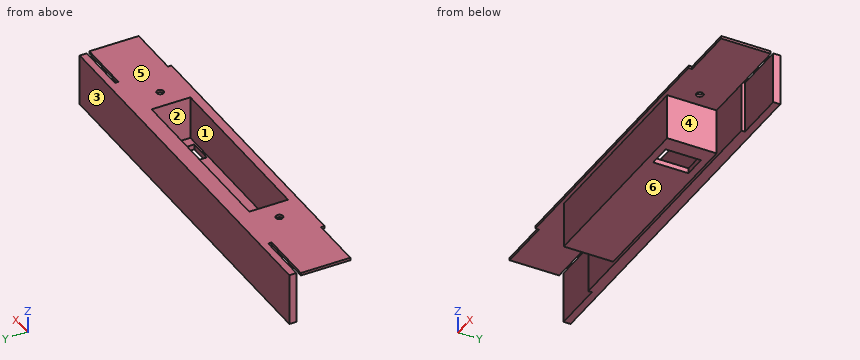
Autodesk Inventor part; units mm, degrees
ref_plane "YZ Plane" through (0, 0, 0) normal (1, 0, 0) x (0, 1, 0)
ref_plane "XZ Plane" through (0, 0, 0) normal (0, 1, 0) x (-1, 0, 0)
ref_plane "XY Plane" through (0, 0, 0) normal (0, 0, 1) x (1, 0, 0)
sketch "Эскиз1" plane through (0, 0, 0) normal (0, 0, 1) x (1, 0, 0)
  line L0 (-54, -14) -> (54, -14)
  line L1 (54, -14) -> (54, 14)
  line L2 (54, 14) -> (-54, 14)
  line L3 (-54, 14) -> (-54, -14)
  line L4 (-54, -14) -> (54, 14) construction
  line L5 (54, -14) -> (-54, 14) construction
  point P0 (0, 0)
  dimension "d0" = 108
  dimension "d1" = 28
extrude "Выдавливание1" add sketch "Эскиз1" along normal blind 27.5
sketch "Эскиз2" plane through (0, 0, 27.5) normal (0, 0, 1) x (1, 0, 0)
  line L0 (-51, -11) -> (51, -11)
  line L1 (51, -11) -> (51, 11)
  line L2 (51, 11) -> (-51, 11)
  line L3 (-51, 11) -> (-51, -11)
  line L4 (-51, -11) -> (51, 11) construction
  line L5 (51, -11) -> (-51, 11) construction
  line L6 (54, 14) -> (-54, 14)
  line L7 (54, -14) -> (54, 14)
  point P0 (0, 0)
  dimension "d4" = 3
  dimension "d5" = 3
extrude "Выдавливание2" cut sketch "Эскиз2" against normal blind 24.5
sketch "Эскиз3" plane through (54, -14, 0) normal (1, 0, 0) x (0, 0, -1)
  line L0 (0, 28) -> (-27.5, 28)
  line L1 (0, 0) -> (-27.5, 0)
  line L2 (-27.5, 28) -> (-26, 28)
  line L3 (-26, 28) -> (-26, 0)
  line L4 (-26, 0) -> (-27.5, 0)
  line L5 (-27.5, 0) -> (-27.5, 28)
  point P0 (0, 14)
  dimension "d8" = 1.5
extrude "Выдавливание3" add sketch "Эскиз3" along normal blind 50
mirror "Зеркальное отражение1" about plane through (0, 0, 0) normal (1, 0, 0) of "Выдавливание3"
move faces "Перенос1" translate (6.5, 0, 0) faces at (104, 4.6667, 27)
move faces "Перенос2" translate (-6.5, 0, 0) faces at (-104, 4.6667, 27)
sketch "Эскиз7" plane through (-54, -14, 0) normal (0, -1, 0) x (1, 0, 0)
  line L0 (-56.5, 27.5) -> (164.5, 27.5)
  line L1 (0, 26) -> (-56.5, 26)
  line L2 (134, 27.5) -> (-26, 27.5)
  line L3 (-26, 27.5) -> (-26, 26)
  line L4 (-26, 26) -> (134, 26)
  line L5 (134, 26) -> (134, 27.5)
  line L6 (0, 0) -> (108, 0)
  point P0 (54, 0)
  point P1 (-26, 26.75)
  point P2 (54, 0)
  dimension "d29" = 160
  dimension "d30" = 80
extrude "Выдавливание7" add sketch "Эскиз7" along normal blind 2
sketch "Эскиз8" plane through (-54, 14, 0) normal (0, 1, 0) x (1, 0, 0)
  line L0 (-56.5, -27.5) -> (164.5, -27.5)
  line L1 (-26, -27.5) -> (134, -27.5)
  line L2 (134, -27.5) -> (134, 2)
  line L3 (134, 2) -> (-26, 2)
  line L4 (-26, 2) -> (-26, -27.5)
  line L5 (108, 0) -> (0, 0)
  point P0 (54, 0)
  point P1 (54, 0)
  dimension "d33" = 160
  dimension "d34" = 80
  dimension "d35" = 29.5
extrude "Выдавливание8" add sketch "Эскиз8" along normal blind 6
sketch "Эскиз9" plane through (80, 14, 26) normal (1, 0, 0) x (0, 0, -1)
  line L0 (28, 0) -> (28, 6)
  line L1 (28, 6) -> (-1.5, 6)
  line L2 (-1.5, 6) -> (-1.5, 2)
  line L3 (-1.5, 2) -> (28, 2)
  line L4 (28, 2) -> (28, 6)
  point P0 (26, -14)
  dimension "d38" = 4
extrude "Выдавливание9" add sketch "Эскиз9" along normal blind 29.5
mirror "Зеркальное отражение3" about plane through (0, 0, 0) normal (1, 0, 0) of "Выдавливание9"
sketch "Эскиз10" plane through (0, 0, 27.5) normal (0, 0, 1) x (1, 0, 0)
  circle A0 centre (-62.25, 0) radius 2
  circle A1 centre (62.25, 0) radius 2
  point P0 (0, 0)
extrude "Выдавливание10" cut sketch "Эскиз10" against normal through all
sketch "Эскиз11" plane through (0, 0, 3) normal (0, 0, 1) x (1, 0, 0)
  line L0 (32, -10) -> (45, -10)
  line L1 (45, -10) -> (45, 10)
  line L2 (45, 10) -> (32, 10)
  line L3 (32, 10) -> (32, -10)
  line L4 (32, -10) -> (45, 10) construction
  line L5 (45, -10) -> (32, 10) construction
  line L6 (51, 11) -> (51, -11)
  point P0 (0, 0)
  point P1 (38.5, 0)
  dimension "d43" = 13
  dimension "d44" = 20
  dimension "d45" = 6
extrude "Выдавливание11" cut sketch "Эскиз11" against normal through all
properties part number "000.009 - Короб" material "Пластик АБС"
Check sheet for the modelled part. Datum: model origin and axes. Units: mm. Face numbers are marked on the shaded views. A direction names the side the tool comes from. Give positions to 0.01 mm unless a question says otherwise; leave off trailing zeros. Order: outer loops, then holes, each group sorted by start corner. A loop starts at its lowest first (then second) coordinate and runs counter-clockwise, first axis right, second up. Notation, with made-up numbers: (75, -15) -> (105, -15) arc R21 cw to (105, 24) -> close; hole circle Ø5 at (84.5, 2.25). An arc over 180 degrees is marked (long way). Use CSV: the item, a comma, the result in double quotes. Start each with the question number.
1) Material ranges on line 1 (Y direction, x = 39, z = 16.5); line 2 (Y direction, x = 62.25, z = 26.65); line 3 (X direction, y = 5.5, z = 8.5), recorded low to high. Write a range as from..to.
2) Sectioned sample at C-C, the plane z = 11.25. Record the boundary of the cut face in (x, y), plus the area to 3 significant figures.
3) Sectioned sample at A-A, the plane y = 0. Record the boundary of the cut face in (x, z).
4) Go/stop test with flat-tipped pins: P1, Ø8.5, axis at x = 19, y = -1.5, coming from the -Z side; P2, Ø4, axis at x = 7.5, z = 3, coming from the -Y side; P3, Ø1.2, axis at y = 19, z = 12.5, coming from the +X side. Record where each tip stops, or that it passes through.
5) Mould release check, pull along Y, two halves, no side actions. Record for the marked faces 1, 2, 3 and 4: released by +Y, released by -Y, zero draft, split by the parting line, or undercut.
6) Sectioned sample at D-D, the plane x = 15. Record the boundary of the cut face in (y, z), plus the area to 3 significant figures.
7) Sectioned sample at B-B, the plane x = 62.25. Record the boundary of the cut face in (y, z), plus the area to 3 significant figures.
8) Set-up check for the marked faces 5 and 6: record each of +Z, -Z, +X, -X, +Y, -Y from which the full face is reachable in a straight line by a thin tool's end or side.
Recorded:
1,line 1,"-14..-11, 11..20"
1,line 2,"-16..-2, 2..20"
1,line 3,"-54..-51, 51..54"
2,outline,"(-109.5, 16) -> (-80, 16) -> (-80, 14) -> (-54, 14) -> (-54, -14) -> (54, -14) -> (54, 14) -> (80, 14) -> (80, 16) -> (109.5, 16) -> (109.5, 20) -> (-109.5, 20) -> close; hole (-51, -11) -> (51, -11) -> (51, 11) -> (-51, 11) -> close"
2,area,"1,980 mm2"
3,outline,"(-110.5, 26) -> (-64.25, 26) -> (-64.25, 27.5) -> (-110.5, 27.5) -> close; (-60.25, 26) -> (-54, 26) -> (-54, 0) -> (32, 0) -> (32, 3) -> (-51, 3) -> (-51, 27.5) -> (-60.25, 27.5) -> close; (45, 0) -> (54, 0) -> (54, 26) -> (60.25, 26) -> (60.25, 27.5) -> (51, 27.5) -> (51, 3) -> (45, 3) -> close; (64.25, 26) -> (110.5, 26) -> (110.5, 27.5) -> (64.25, 27.5) -> close"
4,P1,"z = 0"
4,P2,"y = -14"
4,P3,"x = 109.5"
5,face 1,"undercut"
5,face 2,"undercut"
5,face 3,"released by +Y"
5,face 4,"zero draft"
6,outline,"(-16, 26) -> (-14, 26) -> (-14, 0) -> (14, 0) -> (14, -2) -> (20, -2) -> (20, 27.5) -> (11, 27.5) -> (11, 3) -> (-11, 3) -> (-11, 27.5) -> (-16, 27.5) -> close"
6,area,"411 mm2"
7,outline,"(-16, 26) -> (-2, 26) -> (-2, 27.5) -> (-16, 27.5) -> close; (2, 26) -> (14, 26) -> (14, -2) -> (20, -2) -> (20, 27.5) -> (2, 27.5) -> close"
7,area,"216 mm2"
8,face 5,"+Z, +X, -X, +Y, -Y"
8,face 6,"-Z, +X, -X, -Y"
